Autodesk Inventor part; units mm, degrees
ref_plane "YZ Plane" through (0, 0, 0) normal (1, 0, 0) x (0, 1, 0)
ref_plane "XZ Plane" through (0, 0, 0) normal (0, 1, 0) x (-1, 0, 0)
ref_plane "XY Plane" through (0, 0, 0) normal (0, 0, 1) x (1, 0, 0)
sketch "Sketch1" plane through (0, 0, 0) normal (0, 0, 1) x (1, 0, 0)
  line L0 (0, 0) -> (100, 0)
  line L1 (100, 0) -> (100, -75)
  line L2 (100, -75) -> (75, -118.3013)
  line L3 (-12.5, -50) -> (-12.5, -118.3013)
  arc A0 (0, 0) -> (-12.5, -50) centre (77.4072, -45.9143) ccw
  line L4 (-12.5, -118.3013) -> (75, -118.3013)
  dimension "d0" = 100
  dimension "d1" = 75
  dimension "d2" = 50
  dimension "d3" = 150
  dimension "d4" = 12.5
  dimension "d5" = 50
  dimension "d6" = 90
extrude "Extrusion1" add sketch "Sketch1" along normal blind 50
sketch "Sketch2" plane through (0, 0, 50) normal (0, 0, 1) x (1, 0, 0)
  line L0 (100, 0) -> (0, 0)
  arc A0 (0, 0) -> (-12.5, -50) centre (77.4072, -45.9143) ccw
  line L1 (-12.5, -50) -> (-12.5, -118.3013)
  line L2 (-12.5, -118.3013) -> (75, -118.3013)
  line L3 (75, -118.3013) -> (100, -75)
  line L4 (100, -75) -> (100, 0)
  arc A1 (2.902, -5) -> (-7.5, -49.8848) centre (77.4072, -45.9143) ccw
  line L5 (2.902, -5) -> (95, -5)
  line L6 (95, -5) -> (95, -73.6603)
  line L7 (95, -73.6603) -> (72.1132, -113.3013)
  line L8 (72.1132, -113.3013) -> (-7.5, -113.3013)
  line L9 (-7.5, -113.3013) -> (-7.5, -49.8848)
  dimension "d9" = 5
extrude "Extrusion2" cut sketch "Sketch2" against normal blind 45 contours L5 L6 L7 L8 L9 A1
sketch "Sketch3" plane through (0, 0, 50) normal (0, 0, 1) x (1, 0, 0)
  line L0 (72.1132, -113.3013) -> (-7.5, -113.3013)
  line L1 (-12.5, -118.3013) -> (75, -118.3013)
  line L2 (-7.5, -113.3013) -> (60, -113.3013)
  line L3 (60, -113.3013) -> (60, -118.3013)
  line L4 (60, -118.3013) -> (-7.5, -118.3013)
  line L5 (-7.5, -118.3013) -> (-7.5, -113.3013)
  point P0 (0, 0)
  dimension "d13" = 15
extrude "Extrusion3" cut sketch "Sketch3" against normal blind 45
sketch "Sketch4" plane through (0, 0, 0) normal (0, 1, 0) x (1, 0, 0)
  circle A0 centre (50, -50) radius 6
  line L0 (100, -50) -> (0, -50)
  point P0 (0, 0)
  dimension "d16" = 12
extrude "Extrusion4" cut sketch "Sketch4" against normal through all
sketch "Sketch5" plane through (0, 0, 0) normal (0, 1, 0) x (1, 0, 0)
  arc A0 (56, -50) -> (44, -50) centre (50, -50) ccw
  circle A1 centre (50, -50) radius 30 construction
  circle A2 centre (50, -20) radius 2.5
  circle A3 centre (24.0192, -35) radius 2.5
  circle A4 centre (24.0192, -65) radius 2.5
  circle A5 centre (50, -80) radius 2.5
  circle A6 centre (75.9808, -65) radius 2.5
  circle A7 centre (75.9808, -35) radius 2.5
  point P0 (0, 0)
  dimension "d20" = 60
  dimension "d21" = 5
  dimension "d24" = 360
extrude "Extrusion5" cut sketch "Sketch5" against normal blind 5 contours A2 | A3 | A7
sketch "Sketch6" plane through (0, 0, 50) normal (0, 0, 1) x (1, 0, 0)
  line L0 (-7.5, -113.3013) -> (37.5, -113.3013)
  line L1 (37.5, -113.3013) -> (37.5, -68.3013)
  line L2 (37.5, -68.3013) -> (-7.5, -68.3013)
  line L3 (-7.5, -68.3013) -> (-7.5, -113.3013)
  circle A0 centre (15, -90.8013) radius 2.75
  line L4 (-0.5, -106.3013) -> (30.5, -106.3013) construction
  line L5 (30.5, -106.3013) -> (30.5, -75.3013) construction
  line L6 (30.5, -75.3013) -> (-0.5, -75.3013) construction
  line L7 (-0.5, -75.3013) -> (-0.5, -106.3013) construction
  line L8 (-0.5, -106.3013) -> (30.5, -75.3013) construction
  line L9 (30.5, -106.3013) -> (-0.5, -75.3013) construction
  circle A1 centre (30.5, -75.3013) radius 1.5
  circle A2 centre (-0.5, -75.3013) radius 1.5
  circle A3 centre (-0.5, -106.3013) radius 1.5
  circle A4 centre (30.5, -106.3013) radius 1.5
  point P0 (0, 0)
  point P1 (15, -90.8013)
  point P2 (15, -68.3013)
  point P3 (15, -90.8013)
  point P4 (37.5, -90.8013)
  point P5 (-7.5, -118.3013)
  dimension "d29" = 45
  dimension "d30" = 45
  dimension "d31" = 5.5
  dimension "d32" = 31
  dimension "d33" = 31
  dimension "d34" = 3
  dimension "d35" = 3
  dimension "d36" = 3
  dimension "d37" = 3
  dimension "d61" = 5
extrude "Extrusion6" add sketch "Sketch6" against normal blind 5
sketch "Sketch7" plane through (0, 0, 50) normal (0, 0, 1) x (1, 0, 0)
  circle A0 centre (15, -90.8013) radius 2.75
  circle A1 centre (15, -90.8013) radius 12.5
  point P0 (0, 0)
  dimension "d40" = 25
extrude "Extrusion7" cut sketch "Sketch7" against normal blind 2
sketch "Sketch8" plane through (-7.5, -68.3013, 50) normal (0, 1, 0) x (1, 0, 0)
  line L0 (45, 0) -> (45, 5)
  line L1 (82.5, 50) -> (-5, 50)
  line L2 (45, 0) -> (-5, 0)
  line L3 (-5, 0) -> (-5, 50)
  line L4 (-5, 50) -> (45, 50)
  line L5 (45, 50) -> (45, 0)
  point P0 (7.5, 50)
extrude "Extrusion8" add sketch "Sketch8" along normal blind 5
sketch "Sketch10" plane through (-12.5, -118.3013, 0) normal (0, -1, 0) x (1, 0, 0)
  line L0 (87.5, 0) -> (87.5, 50)
  line L1 (87.5, 0) -> (0, 0)
  line L2 (87.5, 0) -> (32.5, 0)
  line L3 (32.5, 0) -> (32.5, 15)
  line L4 (32.5, 15) -> (87.5, 15)
  line L5 (87.5, 15) -> (87.5, 0)
  line L6 (0, 0) -> (0, 50)
  point P0 (12.5, 0)
  dimension "d49" = 15
  dimension "d50" = 32.5
extrude "Extrusion10" add sketch "Sketch10" against normal blind 5
sketch "Sketch14" plane through (0, 0, 0) normal (0, 0, -1) x (-1, 0, 0)
  circle A0 centre (-15, -90.8013) radius 2.75
  circle A1 centre (0.5, -75.3013) radius 1.5
  circle A2 centre (0.5, -106.3013) radius 1.5
  circle A3 centre (-30.5, -106.3013) radius 1.5
  circle A4 centre (-30.5, -75.3013) radius 1.5
  point P0 (0, 0)
extrude "Extrusion13" cut sketch "Sketch14" against normal through all contours A1 | A2 | A3 | A4
sketch "Sketch15" plane through (0, 0, 5) normal (0, 0, 1) x (1, 0, 0)
  line L0 (20, -113.3013) -> (60, -113.3013)
  line L1 (37.5, -63.3013) -> (42.5, -63.3013)
  line L2 (42.5, -63.3013) -> (42.5, -113.3013)
  line L3 (42.5, -113.3013) -> (37.5, -113.3013)
  line L4 (37.5, -113.3013) -> (37.5, -63.3013)
  point P0 (0, 0)
  dimension "d62" = 5
extrude "Extrusion14" add sketch "Sketch15" along normal blind 45
sketch "Sketch16" plane through (0, 0, 5) normal (0, 0, 1) x (1, 0, 0)
  circle A0 centre (15, -90.8013) radius 10
  point P0 (0, 0)
  dimension "d65" = 20
extrude "Extrusion15" add sketch "Sketch16" along normal blind 15
properties part number "FA001" material "ABS Plastic"
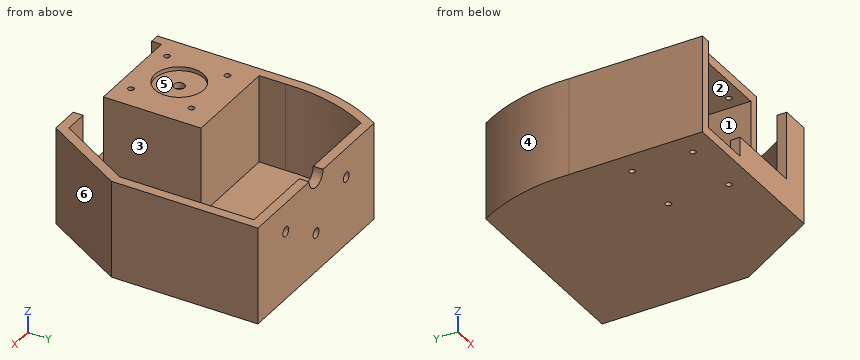
The model under review builds one solid part; all positions refer to its coordinate system, in mm. Face numbers are marked on the shaded views. A direction names the side the tool comes from. Coordinates: 2 decimals unless noted, no trailing zeros. Loops run counter-clockwise (first coordinate to the right, second up) from the corner with the lowest first, then second, coordinate; pieces in that order, holes last. Notation, with made-up numbers: (81.5, 52.5) -> (122.5, 52.5) arc R7 ccw to (122.5, 63.5) -> close; hole circle Ø4 at (86.5, 33). An arc over 180 degrees is marked (long way). Use a Markdown table: item, result. Add a question column.
1. Machinability: for the marked faces 1, 2 and 3, which of the approach directions +Z, -Z, +X, -X, +Y, -Y give a long, thin tool a straight path to every point of the face, cutting with its end or side? Answer none if there is none.
2. Draft analysis for pull direction X (two halves, no side actions). For the marked faces 4, 5 and 6, state which applies: pulls with the +X half, pulls with the -X half, needs draft (parallel to the pull), parting line crosses it, or undercut.
3. To check wall thickness, follow line 1 (Y direction, x = 30.5, z = 48); line 2 (Y direction, x = 41, z = 6.5); line 3 (X direction, y = -93, z = 12). State the ranges of each line that lie inside material, in increasing order.
4. Clearance check with flat-ended pins moving along their axes: pin 1 Ø1.5 at (x, y) = (27, -47) entering from +Z; pin 2 Ø22.5 at (y, z) = (-29, 23) entering from -X; pin 3 Ø3 at (x, z) = (75.98, 35) entering from +Y; pin 4 Ø12 at (x, z) = (11.5, 8) entering from -Y. State where each tip first meets the part, or that it passes through.
5. Add section D-D on y = -109.5. Write out the cut boundary in (x, z), plus the area to 3 significant figures.
6. Add section C-C on z = 7. Write out the cut boundary in (x, y).
7. Add section B-B on x = 15. Write out the cut boundary in (y, z).
8. Add section A-A on x = 30.5. Give the number of separate pieces and of enclosed holes in the cut face, plus the area to 3 significant figures.
Returned:
| question | item | result |
|---|---|---|
| 1 | face 1 | none |
| 1 | face 2 | -Y |
| 1 | face 3 | +Z |
| 2 | face 4 | pulls with the -X half |
| 2 | face 5 | undercut |
| 2 | face 6 | pulls with the +X half |
| 3 | line 1 | y = -113.3 to -107.8, -104.8 to -76.8, -73.8 to -63.3, -5 to 0 |
| 3 | line 2 | y = -118.3 to -63.3, -5 to 0 |
| 3 | line 3 | x = -12.5 to -7.5, 5.24 to 24.76, 37.5 to 42.5, 83.83 to 89.61 |
| 4 | pin 1 | stops at z = 5 |
| 4 | pin 2 | stops at x = -12.41 |
| 4 | pin 3 | stops at y = -104.01 |
| 4 | pin 4 | stops at y = -118.3 |
| 5 | outline | (-12.5, 0) -> (80.08, 0) -> (80.08, 50) -> (74.31, 50) -> (74.31, 5) -> (42.5, 5) -> (42.5, 50) -> (-12.5, 50) -> close; hole (-7.5, 5) -> (37.5, 5) -> (37.5, 45) -> (-7.5, 45) -> close |
| 5 | area | 1,400 mm² |
| 6 | outline | (-12.5, -118.3) -> (-7.5, -118.3) -> (-7.5, -68.3) -> (37.5, -68.3) -> (37.5, -113.3) -> (20, -113.3) -> (20, -118.3) -> (75, -118.3) -> (100, -75) -> (100, 0) -> (0, 0) arc R90 ccw to (-12.5, -50) -> close; circle Ø20 at (15, -90.8); hole (-7.5, -63.3) -> (42.5, -63.3) -> (42.5, -113.3) -> (72.11, -113.3) -> (95, -73.66) -> (95, -5) -> (2.9, -5) arc R85 ccw to (-7.5, -49.88) -> close |
| 7 | outline | (-118.3, 0) -> (0, 0) -> (0, 50) -> (-5, 50) -> (-5, 5) -> (-63.3, 5) -> (-63.3, 50) -> (-78.3, 50) -> (-78.3, 48) -> (-88.05, 48) -> (-88.05, 45) -> (-68.3, 45) -> (-68.3, 5) -> (-80.8, 5) -> (-80.8, 20) -> (-100.8, 20) -> (-100.8, 5) -> (-118.3, 5) -> close; (-113.3, 45) -> (-93.55, 45) -> (-93.55, 48) -> (-103.3, 48) -> (-103.3, 50) -> (-113.3, 50) -> close |
| 8 | separate pieces | 5 |
| 8 | enclosed holes | 0 |
| 8 | area | 1,260 mm² |
